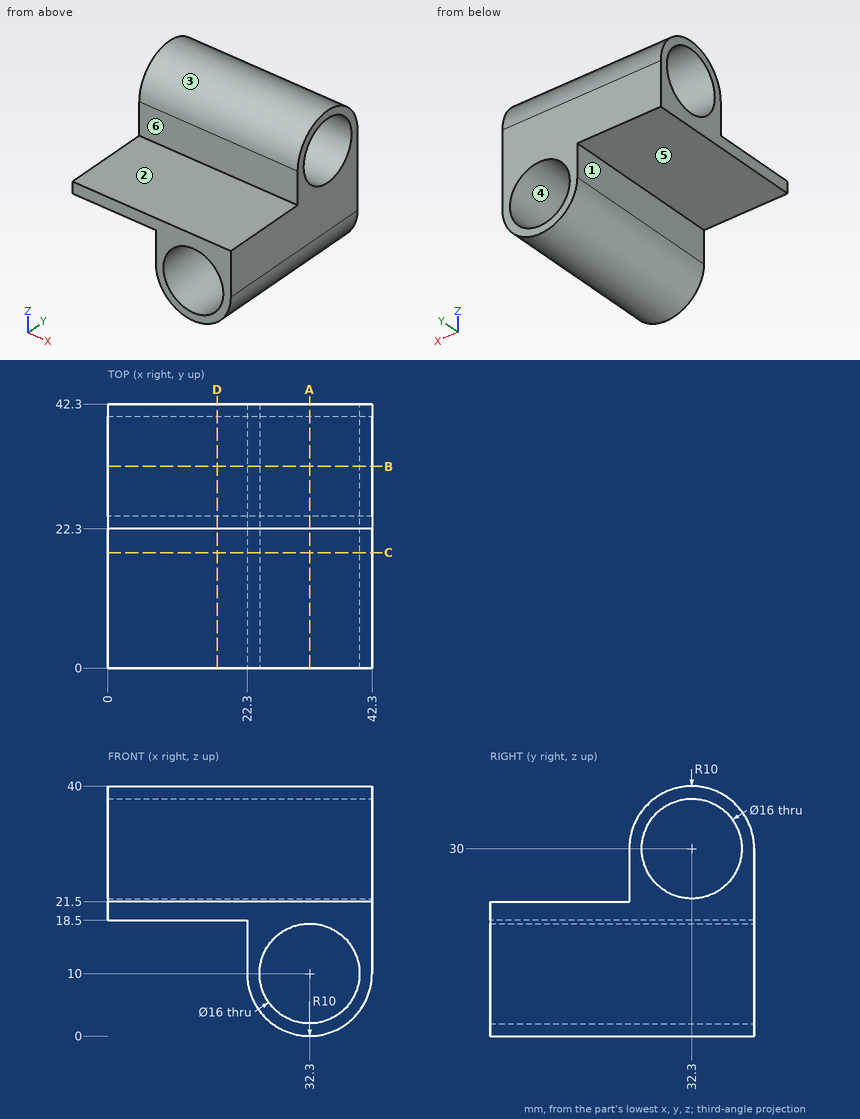
Geometry check sheet. Reference: drawing and pictorial views, mm from the part's lowest x, y, z. A direction names the side the tool comes from. Round coordinates to 2 decimals unless told otherwise and drop trailing zeros. Loops run counter-clockwise (first coordinate to the right, second up) from the corner with the lowest first, then second, coordinate; pieces in that order, holes last.
1. Sectioned sample at A-A on x = 32.3. Record the boundary of the cut face in (y, z).
2. Sectioned sample at C-C on y = 18.5. Record the boundary of the cut face in (x, z), and give its area (3 significant figures).
3. Mould release check, pull along Z, two halves, no side actions. Record for the marked faces 4, 5 and 6: released by +Z, released by -Z, zero draft, split by the parting line, or undercut.
4. Sectioned sample at D-D on x = 17.5. Record the boundary of the cut face in (y, z).
5. Gauge pin test, flat ends, axial feed: pin 1 Ø2 at (x, y) = (11, 36) entering from -Z; pin 2 Ø4 at (y, z) = (24.5, 13) entering from -X; pin 3 Ø10 at (x, y) = (34.5, 22.5) entering from -Z; pin 4 Ø2 at (x, z) = (9, 33) entering from +Y. Record the tip position at first contact, or that the pin passes through.
6. Set-up check for the marked faces 1, 2 and 3: record each of +Z, -Z, +X, -X, +Y, -Y from which the full face is reachable in a straight line by a thin tool's end or side.
7. Sectioned sample at B-B on y = 32.3. Record the boundary of the cut face in (x, z).
8. Scan lines: probe 1 along Z at (x, y) = (32.3, 25); probe 2 along Z at (x, y) = (32.3, 19); probe 3 along Z at (x, y) = (32, 27). Record each from-to range of solid material in increasing order.
Recorded:
1. outline: (0, 0) - (42.3, 0) - (42.3, 2) - (0, 2) - close; (0, 18) - (42.3, 18) - (42.3, 30) arc R10 ccw to (22.3, 30) - (22.3, 21.5) - (0, 21.5) - close; hole circle Ø16 at (32.3, 30)
2. outline: (0, 18.5) - (22.3, 18.5) - (22.3, 10) arc R10 ccw to (42.3, 10) - (42.3, 21.5) - (0, 21.5) - close; hole circle Ø16 at (32.3, 10)
2. area: 253 mm2
3. face 4: undercut
3. face 5: released by -Z
3. face 6: zero draft
4. outline: (0, 18.5) - (42.3, 18.5) - (42.3, 30) arc R10 ccw to (22.3, 30) - (22.3, 21.5) - (0, 21.5) - close; hole circle Ø16 at (32.3, 30)
5. pin 1: stops at z = 18.5
5. pin 2: stops at x = 22.3
5. pin 3: stops at z = 0
5. pin 4: stops at y = 42.1
6. face 1: -Z, -X, +Y, -Y
6. face 2: +Z, +X, -X, -Y
6. face 3: +Z, +X, -X
7. outline: (0, 18.5) - (22.3, 18.5) - (22.3, 10) arc R10 ccw to (42.3, 10) - (42.3, 22) - (0, 22) - close; (0, 38) - (42.3, 38) - (42.3, 40) - (0, 40) - close; hole circle Ø16 at (32.3, 10)
8. probe 1: z = 0 to 2, 18 to 26.73, 33.27 to 36.83
8. probe 2: z = 0 to 2, 18 to 21.5
8. probe 3: z = 0 to 2.01, 17.99 to 24.01, 35.99 to 38.48
